Source: three-view drawing plus pictorial views. Frame: mm from the lowest corner of the part. Round coordinates to 2 decimals unless told otherwise and drop trailing zeros. Loops run counter-clockwise (first coordinate to the right, second up) from the corner with the lowest first, then second, coordinate; pieces in that order, holes last. Notation, with made-up numbers: (44.5, -9.5) -> (85.5, -9.5) arc R25 ccw to (85.5, 12.5) -> close; hole circle Ø9 at (57, 50). An arc over 180 degrees is marked (long way). Answer as a JSON object with one key per item and string values. Group by question number.
Item 1: Section query B-B on x = 45. Return loops of the section in (y, z) (1 decimal).
Item 2: Section query A-A on x = 77. Return loops of the section in (y, z).
Item 3: Material intervals for line 1 (Z direction, x = 76, y = 75); line 2 (Y direction, x = 46, z = 9) (1 decimal), sorted ascending. Write a range as [from, to].
Item 4: Pin query (flat end, axial travel): pin 1 (3.5 mm diameter, centred on x = 73.5, y = 71, fed in from +Z). Return the tip coordinate at first contact, or that it passes through.
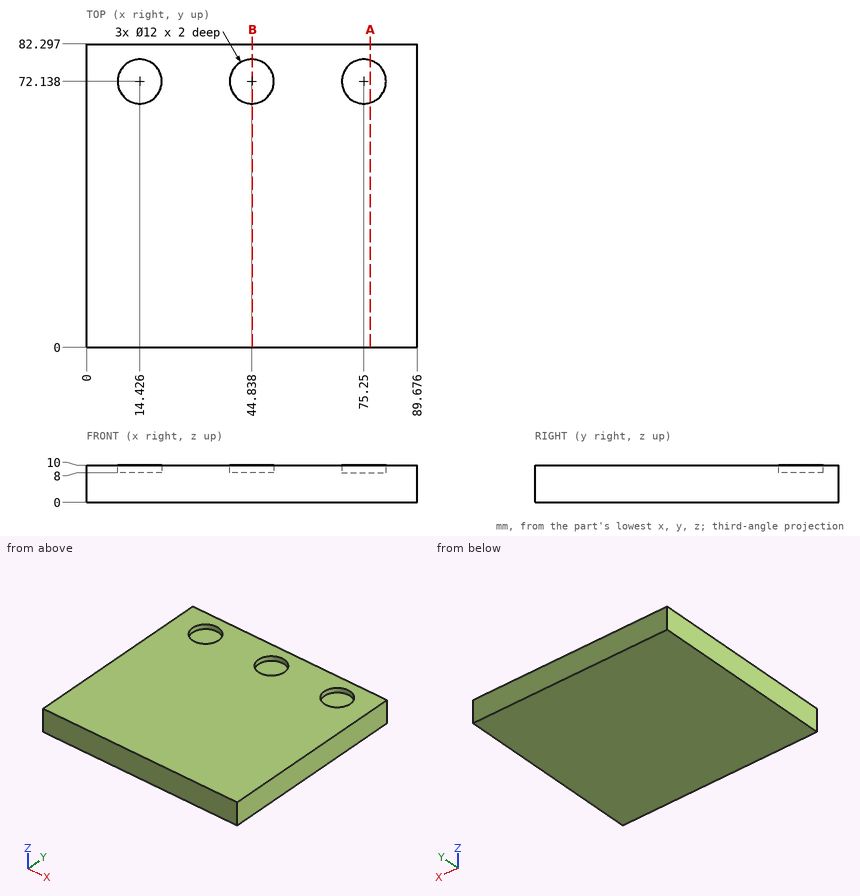
Solved:
{
 "1": {"outline": "(0, 0) -> (82.3, 0) -> (82.3, 10) -> (78.1, 10) -> (78.1, 8) -> (66.1, 8) -> (66.1, 10) -> (0, 10) -> close"},
 "2": {"outline": "(0, 0) -> (82.3, 0) -> (82.3, 10) -> (77.88, 10) -> (77.88, 8) -> (66.4, 8) -> (66.4, 10) -> (0, 10) -> close"},
 "3": {"line 1": "[0, 8]", "line 2": "[0, 66.3], [78, 82.3]"},
 "4": {"pin 1": "z = 8"}
}
